The figure shows three views and two pictorial views of one solid part (mm, origin at its lowest corner). Answer the questions. A direction names the side the tool comes from. Coordinates: 2 decimals unless noted, no trailing zeros. Loops run counter-clockwise (first coordinate to the right, second up) from the corner with the lowest first, then second, coordinate; pieces in that order, holes last. Notation, with made-up numbers: (-33, 53) - (-2, 53) arc R18 ccw to (-2, 83) - close; hole circle Ø6 at (78, 24.5). An arc over 180 degrees is marked (long way). One line per question, with ' | ' between items.
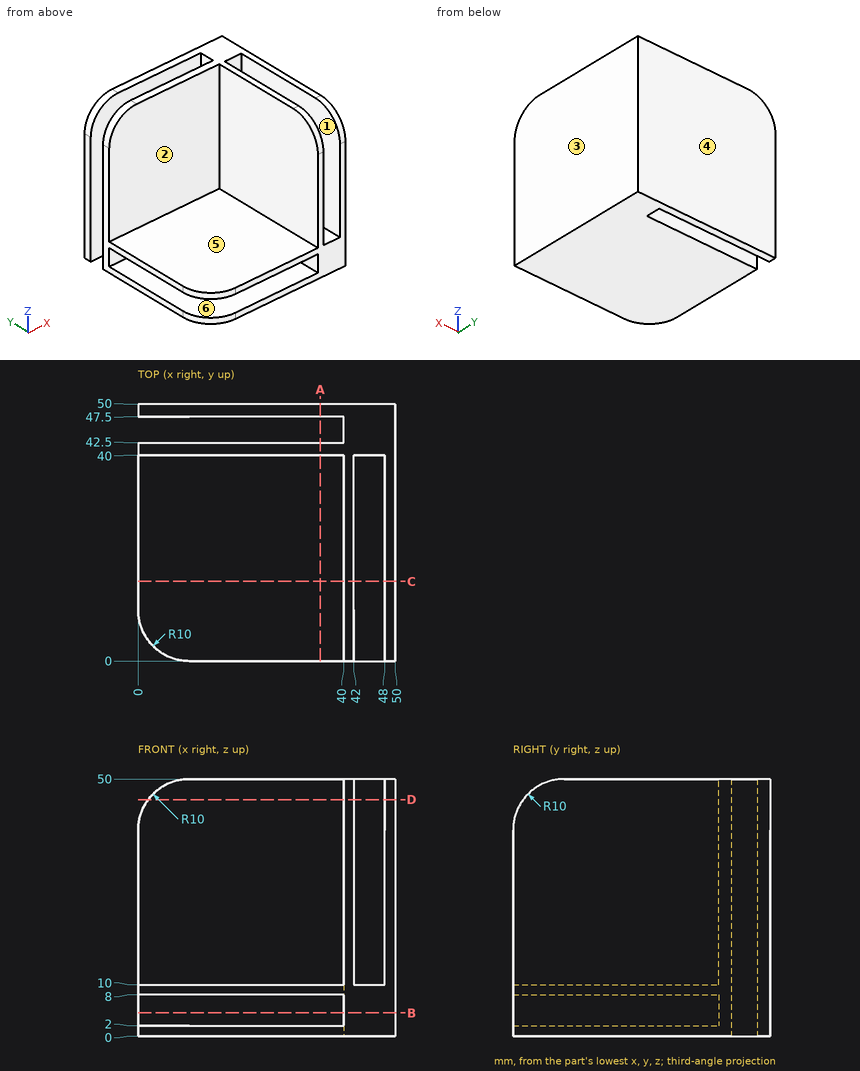
Item 1: Which of the six approach directions +Z, -Z, +X, -X, +Y, -Y give full straight-line access (tool end or side, diameter ignored) to the marked faces 4, 5 and 6?
Taken from the geometry:
face 4: +Z, -Z, +X, -X, +Y | face 5: +Z, -X, -Y | face 6: -X, -Y
Item 2: Find section A-A, the plane x = 35.5. Write down the section's boundary in (y, z).
Taken from the geometry:
outline: (0, 0) - (42.5, 0) - (42.5, 50) - (40, 50) - (40, 10) - (0, 10) - (0, 8) - (40, 8) - (40, 2) - (0, 2) - close; (47.5, 0) - (50, 0) - (50, 50) - (47.5, 50) - close
Item 3: Each of these flat-tipped pins is pushed along its axis until it touches: pin 1 Ø12 at (y, z) = (19, 25.5) entering from -X; pin 2 Ø20 at (x, z) = (27.5, 23.5) entering from -Y; pin 3 Ø1 at (x, y) = (15.5, 18.5) entering from +Z. Where does it stop, or does it pass through?
Taken from the geometry:
pin 1: stops at x = 40 | pin 2: stops at y = 40 | pin 3: stops at z = 10
Item 4: Find the intervals of material crossed by line 1 (Y direction, x = 11, z = 28.5); line 2 (X direction, y = 3.5, z = 30); line 3 (Z direction, x = 11, y = 4), in increasing order. Write a range as [from, to].
Taken from the geometry:
line 1: y = [40, 42.5], [47.5, 50] | line 2: x = [40, 42], [48, 50] | line 3: z = [0, 2], [8, 10]
Item 5: Find section C-C, the plane y = 15.5. Write down the section's boundary in (x, z).
Taken from the geometry:
outline: (0, 0) - (50, 0) - (50, 50) - (48, 50) - (48, 10) - (42, 10) - (42, 50) - (40, 50) - (40, 10) - (0, 10) - (0, 8) - (40, 8) - (40, 2) - (0, 2) - close
Item 6: Find section D-D, the plane z = 46. Write down the section's boundary in (x, y), plus the area to 3 significant figures.
Taken from the geometry:
outline: (2, 40) - (40, 40) - (40, 2) - (42, 2) - (42, 40) - (48, 40) - (48, 2) - (50, 2) - (50, 50) - (2, 50) - (2, 47.5) - (40, 47.5) - (40, 42.5) - (2, 42.5) - close | area: 442 mm2
Item 7: Find section B-B, the plane z = 4.5. Write down the section's boundary in (x, y), plus the area to 3 significant figures.
Taken from the geometry:
outline: (0, 40) - (40, 40) - (40, 0) - (50, 0) - (50, 50) - (0, 50) - (0, 47.5) - (40, 47.5) - (40, 42.5) - (0, 42.5) - close | area: 700 mm2
Item 8: The mould has two halves that part along X. Classify the marked faces 1, 2 and 3: pulls with the +X half, pulls with the -X half, needs draft (parallel to the pull), parting line crosses it, or undercut.
Taken from the geometry:
face 1: undercut | face 2: needs draft | face 3: pulls with the +X half
